Study the drawing (mm; zero at the part's minimum x, y, z) and answer. Round coordinates to 2 decimals unless told otherwise and drop trailing zeros. Order: outer loops, then holes, each group sorted by start corner. A loop starts at its lowest first (then second) coordinate and runs counter-clockwise, first axis right, second up. Notation, with made-up numbers: (-33, 36) - (20, 36) arc R12 cw to (20, 42) - close; hole circle Ø11 at (57, 82.25). An arc over 180 degrees is marked (long way). Put each result on its own line as item: value.
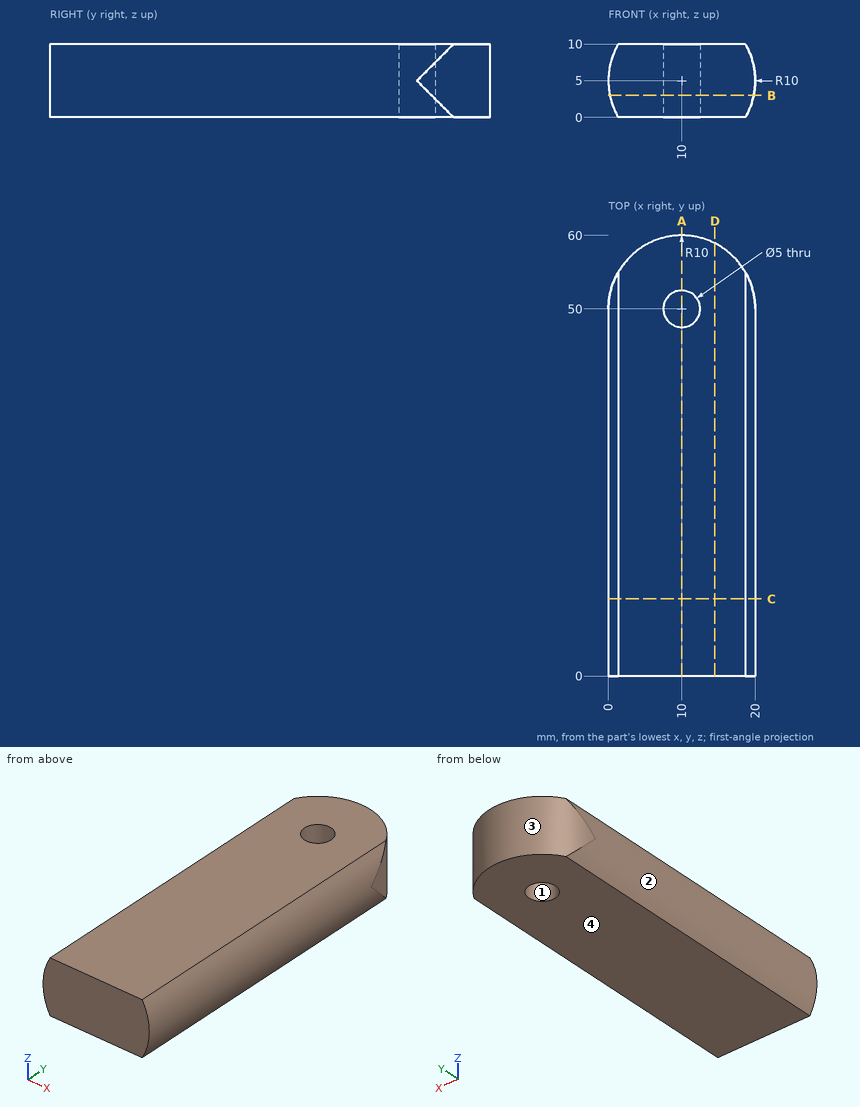
1) Straight lines are drawn through the part: L1, parallel to Y at x = 12, z = 7; L2, parallel to Y at x = 11, z = 4; L3, parallel to Y at x = 14.25, z = 5.5. For each, find the intervals that lie inside material, in ascending order. Write a range as from..to.
Findings below:
L1: y = 0..48.5, 51.5..59.8
L2: y = 0..47.71, 52.29..59.95
L3: y = 0..59.05
2) Given pin 1 Ø2 at (y, z) = (28, 7.5) entering from +X; pin 2 Ø6.5 at (x, y) = (10, 50) entering from +Z, each flat-ended and moving along its own axis, determine where each tip first touches the part or whether it passes through.
Findings below:
pin 1: stops at x = 19.89
pin 2: stops at z = 10
3) A cutting plane is placed at D-D on x = 14.5. Write down the section's boundary in (y, z), then the cut area to 3 significant figures.
Findings below:
outline: (0, 0) - (58.93, 0) - (58.93, 10) - (0, 10) - close
area: 589 mm2
4) For a pull along X with two mould halves and no side action, classify the marked faces 1, 2, 3 and 4 as pulls with the +X half, pulls with the -X half, needs draft (parallel to the pull), parting line crosses it, or undercut.
Findings below:
face 1: undercut
face 2: pulls with the -X half
face 3: parting line crosses it
face 4: needs draft
5) A cutting plane is placed at A-A on x = 10. Write down the section's boundary in (y, z), then the cut area to 3 significant figures.
Findings below:
outline: (0, 0) - (47.5, 0) - (47.5, 10) - (0, 10) - close; (52.5, 0) - (60, 0) - (60, 10) - (52.5, 10) - close
area: 550 mm2
6) A cutting plane is placed at B-B on z = 3. Write down the section's boundary in (x, y), then the cut area to 3 significant figures.
Findings below:
outline: (0.2, 0) - (19.8, 0) - (19.8, 52) arc R10 ccw to (0.2, 52) - close; hole circle Ø5 at (10, 50)
area: 1,120 mm2
7) A cutting plane is placed at C-C on y = 10.5. Write down the section's boundary in (x, z), then the cut area to 3 significant figures.
Findings below:
outline: (1.34, 0) - (18.66, 0) arc R10 ccw to (18.66, 10) - (1.34, 10) arc R10 ccw to start
area: 191 mm2
